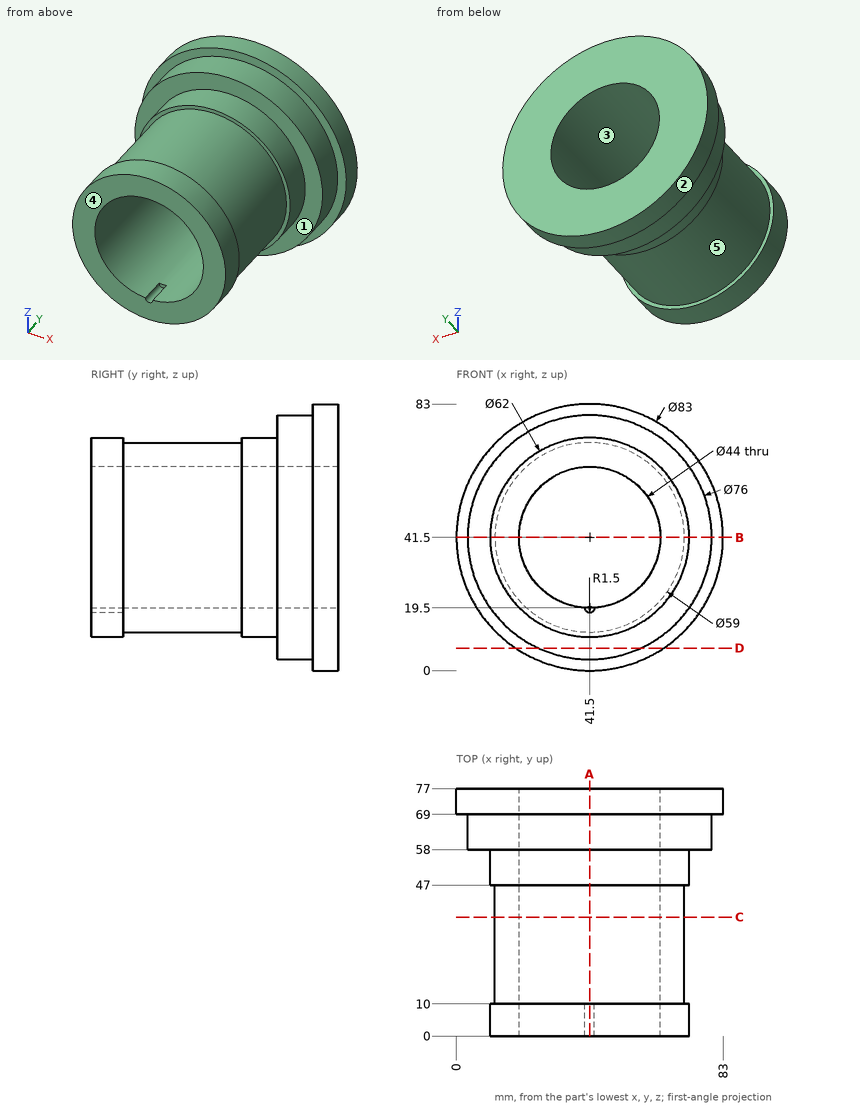
Geometry check sheet. Reference: drawing and pictorial views, mm from the part's lowest x, y, z. A direction names the side the tool comes from. Round coordinates to 2 decimals unless told otherwise and drop trailing zeros. Order: outer loops, then holes, each group sorted by start corner. A loop starts at its lowest first (then second) coordinate and runs counter-clockwise, first axis right, second up. Notation, with made-up numbers: (54, 16) -> (85, 16) arc R18 ccw to (85, 43) -> close; hole circle Ø9 at (-39.75, 80.25). An arc over 180 degrees is marked (long way). One line per item, written item: value. Start each with the question number.
Q1. Set-up check for the marked faces 1 and 2: record each of +Z, -Z, +X, -X, +Y, -Y from which the full face is reachable in a straight line by a thin tool's end or side.
Q2. Cross-section at C-C (y = 37). Record the boundary of the cut face in (x, z), and give its area (3 significant figures).
Q3. Gauge pin test, flat ends, axial feed: pin 1 Ø0.5 at (x, z) = (41.5, 19) entering from -Y; pin 2 Ø4 at (y, z) = (26, 49) entering from +X; pin 3 Ø10 at (x, y) = (69.5, 61.5) entering from -Z. Record the tip position at first contact, or that the pin passes through.
Q4. Thickness scan on line 1 (Z direction, x = 41, y = 18); line 2 (X direction, y = 53.5, z = 41.5); line 3 (X direction, y = 29, z = 41.5). Record the ranges inside material, lowest first.
Q5. Cross-section at B-B (z = 41.5). Record the boundary of the cut face in (x, y), and give its area (3 significant figures).
Q6. Cross-section at A-A (x = 41.5). Record the boundary of the cut face in (y, z).
Q7. Cross-section at D-D (z = 7). Record the boundary of the cut face in (x, y), and give its area (3 significant figures).
Q8. Mould release check, pull along X, two halves, no side actions. Record for the marked faces 3, 4 and 5: pulls with the +X half, pulls with the -X half, needs draft (parallel to the pull), parting line crosses it, or undercut.
Completed:
1. face 1: -Y
1. face 2: +Y, -Y
2. outline: circle Ø59 at (41.5, 41.5); hole circle Ø44 at (41.5, 41.5)
2. area: 1,210 mm²
3. pin 1: stops at y = 10
3. pin 2: stops at x = 70.48
3. pin 3: stops at z = 11.25
4. line 1: z = 12 to 19.51, 63.49 to 71
4. line 2: x = 10.5 to 19.5, 63.5 to 72.5
4. line 3: x = 12 to 19.5, 63.5 to 71
5. outline: (0, 69) -> (3.5, 69) -> (3.5, 58) -> (10.5, 58) -> (10.5, 47) -> (12, 47) -> (12, 10) -> (10.5, 10) -> (10.5, 0) -> (19.5, 0) -> (19.5, 77) -> (0, 77) -> close; (63.5, 0) -> (72.5, 0) -> (72.5, 10) -> (71, 10) -> (71, 47) -> (72.5, 47) -> (72.5, 58) -> (79.5, 58) -> (79.5, 69) -> (83, 69) -> (83, 77) -> (63.5, 77) -> close
5. area: 1,600 mm²
6. outline: (0, 10.5) -> (10, 10.5) -> (10, 12) -> (47, 12) -> (47, 10.5) -> (58, 10.5) -> (58, 3.5) -> (69, 3.5) -> (69, 0) -> (77, 0) -> (77, 19.5) -> (10, 19.5) -> (10, 18) -> (0, 18) -> close; (0, 63.5) -> (77, 63.5) -> (77, 83) -> (69, 83) -> (69, 79.5) -> (58, 79.5) -> (58, 72.5) -> (47, 72.5) -> (47, 71) -> (10, 71) -> (10, 72.5) -> (0, 72.5) -> close
7. outline: (18.43, 69) -> (25.57, 69) -> (25.57, 58) -> (57.43, 58) -> (57.43, 69) -> (64.57, 69) -> (64.57, 77) -> (18.43, 77) -> close
7. area: 719 mm²
8. face 3: undercut
8. face 4: needs draft
8. face 5: parting line crosses it
